```python
from build123d import *

# Parameters (mm, degrees)
SKETCH1_W               = 126
SKETCH1_H               = 15
SKETCH1_R               = 2.4
SKETCH1_R_2             = 2.2
BOSS_EXTRUDE1_DEPTH     = 9
SKETCH2_W               = 18
SKETCH2_H               = 15
BOSS_EXTRUDE2_DEPTH     = 29.15
CUT_EXTRUDE1_DEPTH      = 133.500650942
CUT_EXTRUDE1_DEPTH_BACK = 133.500650942
SKETCH4_R               = 4.075
CUT_EXTRUDE2_DEPTH      = 6.5
CHAMFER1_SIZE           = 2.5


with BuildPart() as part:
    # Sketch1 → Boss-Extrude1 (new body)
    with BuildSketch(Plane.XY):
        with Locations((63, -7.5)):
            Rectangle(SKETCH1_W, SKETCH1_H)
        with Locations((42, -7.5)):
            Circle(SKETCH1_R, mode=Mode.SUBTRACT)
        with Locations((7.5, -7.5)):
            Circle(SKETCH1_R_2, mode=Mode.SUBTRACT)
        with Locations(Location((118.5, -7.5, 0), (0, 0, 180))):
            Circle(SKETCH1_R_2, mode=Mode.SUBTRACT)
        with Locations(Location((84, -7.5, 0), (0, 0, 180))):
            Circle(SKETCH1_R, mode=Mode.SUBTRACT)
    extrude(amount=BOSS_EXTRUDE1_DEPTH)

    # Sketch2 → Boss-Extrude2 (add)
    with BuildSketch(Plane.XY.offset(9)):
        with Locations((101, -7.5)):
            Rectangle(SKETCH2_W, SKETCH2_H)
        with Locations((25, -7.5)):
            Rectangle(SKETCH2_W, SKETCH2_H)
    extrude(amount=BOSS_EXTRUDE2_DEPTH)

    # Sketch4 → Cut-Extrude1 (cut, two sides: drawn at the far end of the back side and taken through both)
    with BuildSketch(Plane.XZ.offset(15).offset(-CUT_EXTRUDE1_DEPTH_BACK)):
        with Locations(Location((25, 29, 0), (0, 0, 270))):
            Circle(SKETCH4_R)
        with Locations(Location((101, 29, 0), (0, 0, 90))):
            Circle(SKETCH4_R)
    extrude(amount=CUT_EXTRUDE1_DEPTH + CUT_EXTRUDE1_DEPTH_BACK, mode=Mode.SUBTRACT)

    # Sketch5 → Cut-Extrude2 (cut)
    with BuildSketch(Plane(origin=(0, 0, 0), x_dir=(-1, 0, 0), z_dir=(0, 0, -1))):
        Polygon((-81.892671517, -11.15), (-79.785343035, -7.5), (-81.892671517, -3.85), (-86.107328483, -3.85), (-88.214656965, -7.5), (-86.107328483, -11.15), align=None)
        Polygon((-39.892671517, -11.15), (-44.107328483, -11.15), (-46.214656965, -7.5), (-44.107328483, -3.85), (-39.892671517, -3.85), (-37.785343035, -7.5), align=None)
    extrude(amount=-CUT_EXTRUDE2_DEPTH, mode=Mode.SUBTRACT)

    # Sketch7 → Cut-Revolve1 (revolve, cut)
    with BuildSketch(Plane(origin=(118.5, 0, 0), x_dir=(0, 0, -1), z_dir=(1, 0, 0)), mode=Mode.PRIVATE) as cut_revolve1_sk:
        Polygon((-9, -7.5), (-6, -7.5), (-6, -5.3), (-9, -2.692139787), align=None)
    cut_revolve1 = revolve(cut_revolve1_sk.sketch.rotate(Axis((118.5, -7.5, 9), (0, 0, -1)), 270), axis=Axis((118.5, -7.5, 9), (0, 0, -1)), mode=Mode.SUBTRACT)

    # Mirror1: Cut-Revolve1 across plane
    add(cut_revolve1.mirror(Plane(origin=(63, 0, 0), x_dir=(0, 0, 1), z_dir=(1, 0, 0))), mode=Mode.SUBTRACT)

    # Chamfer1
    chamfer1_edges = [part.edges().sort_by_distance(p)[0] for p in [
        (34, -7.5, 38.15),
        (16, -7.5, 38.15),
        (110, -7.5, 38.15),
        (92, -7.5, 38.15),
        (0, 0, 4.5),
        (126, 0, 4.5),
        (126, -15, 4.5),
        (0, -15, 4.5),
    ]]
    chamfer(chamfer1_edges, length=CHAMFER1_SIZE)


solid = part.part
```
Geometry: final body of the model. Coordinates: model frame, mm. A direction names the side the tool comes from. Coordinates: 2 decimals unless noted, no trailing zeros. Order: outer loops, then holes, each group sorted by start corner. A loop starts at its lowest first (then second) coordinate and runs counter-clockwise, first axis right, second up. Notation, with made-up numbers: (22.25, 71.5) - (39.25, 71.5) arc R19 ccw to (39.25, 86.5) - close; hole circle Ø9 at (11, -22). An arc over 180 degrees is marked (long way). Return JSON: item names as keys, results as strings. Group by question number.
1. Cut plane D-D (x = 101). Output: boundary loops of the cut face in (y, z) (3 decimals).
2. Pin query (flat end, axial travel): pin 1 (7.5 mm diameter, centred on x = 76, y = -8, fed in from +Z); pin 2 (5 mm diameter, centred on y = -3, z = 12, fed in from -X); pin 3 (1 mm diameter, centred on y = -13, z = 23.5, fed in from +X). Return the tip coordinate at first contact, or that it passes through.
3. Cut plane C-C (z = 27.5). Output: boundary loops of the cut face in (x, y), plus the area to 3 significant figures.
4. Pull-direction query (X, two-part tool) for faces 5 (the face through (108.73, -7.6, 36.92)), 6 (the face through (0, -8, 4)), 7 (the face through (81.783, -6.581, 7.732)), 8 (the face through (101, -7, 38.15)); classes: pulls with the +X half, pulls with the -X half, needs draft (parallel to the pull), parting line crosses it, or undercut.
5. Set-up query: faces 1 (the face through (124.8, -13.7, 4.4)), 2 (the face through (38.824, -9.299, 3.204)), 3 (the face through (16, -8, 22)), 4 (the face through (32.77, -7.6, 36.88)). Return all of +Z, -Z, +X, -X, +Y, -Y with unobstructed straight access to the full face (end or side cutting, diameter ignored); none if empty.
6. Material intervals for line 1 along X through (y, z) = (-4.5, 29) (3 decimals); line 2 along Y through (x, z) = (84, 7.15); line 3 along X through (y, z) = (-4, 24), sorted ascending. Write a range as [from, to].
7. Cut plane A-A (z = 16.5). Output: boundary loops of the cut face in (x, y).
8. Cut plane B-B (x = 7.5). Output: boundary loops of the cut face in (y, z).
Resolved:
{
 "1": {"outline": "(-15, 0) - (0, 0) - (0, 24.925) - (-15, 24.925) - close; (-15, 33.075) - (0, 33.075) - (0, 38.15) - (-15, 38.15) - close"},
 "2": {"pin 1": "stops at z = 9", "pin 2": "stops at x = 16", "pin 3": "stops at x = 110"},
 "3": {"outline": "(16, -15) - (21.21, -15) - (21.21, 0) - (16, 0) - close; (28.79, -15) - (34, -15) - (34, 0) - (28.79, 0) - close; (92, -15) - (97.21, -15) - (97.21, 0) - (92, 0) - close; (104.79, -15) - (110, -15) - (110, 0) - (104.79, 0) - close", "area": "313 mm²"},
 "4": {"face 5": "pulls with the +X half", "face 6": "pulls with the -X half", "face 7": "undercut", "face 8": "needs draft"},
 "5": {"face 1": "+Z, -Z, +X, -Y", "face 2": "-Z", "face 3": "+Z, -X, +Y, -Y", "face 4": "+Z, +Y, -Y"},
 "6": {"line 1": "x = [16, 20.925], [29.075, 34], [92, 96.925], [105.075, 110]", "line 2": "y = [-15, -9.9], [-5.1, 0]", "line 3": "x = [16, 34], [92, 110]"},
 "7": {"outline": "(16, -15) - (34, -15) - (34, 0) - (16, 0) - close; (92, -15) - (110, -15) - (110, 0) - (92, 0) - close"},
 "8": {"outline": "(-15, 0) - (-9.7, 0) - (-9.7, 6) - (-12.31, 9) - (-15, 9) - close; (-5.3, 0) - (0, 0) - (0, 9) - (-2.69, 9) - (-5.3, 6) - close"}
}
